Autodesk Fusion 360 part; units mm, degrees
sketch "Sketch2" plane through (0, 0, 0) normal (1, 0, 0) x (0, 1, 0)
  line L0 (-56.0607, 28.9615) -> (-14.2484, 28.9615)
  line L1 (-9.4019, 28.157) -> (-6.4108, 27.1358)
  arc A0 (-6.4108, 27.1358) -> (-8.6089, 30.3207) centre (-5.3607, 30.2115) ccw
  circle A1 centre (-5.3607, 30.2115) radius 2.75
  line L2 (-56.0607, 26.4615) -> (-14.2484, 26.4615)
  line L3 (-10.2097, 25.791) -> (-7.2185, 24.7698)
  arc A2 (-7.2185, 24.7698) -> (-11.1075, 30.4047) centre (-5.3607, 30.2115) ccw
  line L4 (-56.0607, 28.9615) -> (-56.0607, 26.4615)
  line L5 (-11.1075, 30.4047) -> (-11.1411, 29.4053)
  line L6 (-11.1411, 29.4053) -> (-8.6425, 29.3212)
  line L7 (-8.6425, 29.3212) -> (-8.6089, 30.3207)
  arc A3 (-9.4019, 28.157) -> (-14.2484, 28.9615) centre (-14.2484, 13.9615) ccw
  arc A4 (-10.2097, 25.791) -> (-14.2484, 26.4615) centre (-14.2484, 13.9615) ccw
  line L8 (14.6393, 52.3652) -> (14.6393, 9.6795) construction
  arc A5 (40.386, 30.4047) -> (36.497, 24.7698) centre (34.6393, 30.2115) ccw
  circle A6 centre (34.6393, 30.2115) radius 2.75
  line L9 (85.3393, 28.9615) -> (43.5269, 28.9615)
  line L10 (85.3393, 28.9615) -> (85.3393, 26.4615)
  arc A7 (43.5269, 28.9615) -> (38.6804, 28.157) centre (43.5269, 13.9615) ccw
  line L11 (40.386, 30.4047) -> (40.4196, 29.4053)
  arc A8 (37.8874, 30.3207) -> (35.6893, 27.1358) centre (34.6393, 30.2115) ccw
  line L12 (38.6804, 28.157) -> (35.6893, 27.1358)
  line L13 (40.4196, 29.4053) -> (37.921, 29.3212)
  line L14 (39.4882, 25.791) -> (36.497, 24.7698)
  line L15 (85.3393, 26.4615) -> (43.5269, 26.4615)
  arc A9 (43.5269, 26.4615) -> (39.4882, 25.791) centre (43.5269, 13.9615) ccw
  line L16 (37.921, 29.3212) -> (37.8874, 30.3207)
  dimension "d1" = 5.5
  dimension "d2" = 50.7
  dimension "d3" = 2.5
  dimension "d4" = 0
  dimension "d5" = 0.5
  dimension "d6" = 0
  dimension "d7" = 1
  dimension "d8" = 15
  dimension "d9" = 20
extrude "Extrude1" add sketch "Sketch2" along normal blind 101.4 contours L0 L1 A0 L2 L3 A2 L4 L5 L6 L7 A3 A4
sketch "Sketch1" plane through (0, 0, 28.9615) normal (0, 0, 1) x (-1, 0, 0)
  line L0 (0, 14.2484) -> (0, 56.0607)
  line L1 (0, 56.0607) -> (-101.4, 56.0607)
  line L2 (-101.4, 56.0607) -> (-101.4, 14.2484)
  line L3 (-101.4, 14.2484) -> (0, 14.2484)
  line L4 (0, 14.2484) -> (18.3824, 20.4527)
  line L5 (18.3824, 20.4527) -> (18.3824, -4.9808)
  line L6 (18.3824, -4.9808) -> (-17.5, -4.9808)
  line L7 (-17.5, -4.9808) -> (-17.5, 14.2484)
  line L8 (-40.8, 14.2484) -> (-40.8, 11.0057)
  line L9 (-40.8, 11.0057) -> (-40.8, -4.9808)
  line L10 (-40.8, -4.9808) -> (-60.6, -4.9808)
  line L11 (-60.6, -4.9808) -> (-60.6, 14.2484)
  line L12 (-83.9, 14.2484) -> (-83.9, -4.9808)
  line L13 (-83.9, -4.9808) -> (-134.9138, -4.9808)
  line L14 (-134.9138, -4.9808) -> (-127.3022, 20.8989)
  line L15 (-127.3022, 20.8989) -> (-101.4, 14.2484)
  circle A0 centre (-13.3, 46.0607) radius 3.6
  circle A1 centre (-63.3, 46.0607) radius 3.6
  circle A2 centre (-38.3, 37.0607) radius 3.6
  circle A3 centre (-88.3, 37.0607) radius 3.6
  arc A4 (0, 39.0607) -> (-17, 56.0607) centre (-17, 39.0607) ccw
  arc A5 (-84.4, 56.0607) -> (-101.4, 39.0607) centre (-84.4, 39.0607) ccw
  line L16 (0, 11.1411) -> (0, 8.6425)
  line L17 (-60.6, 11.6411) -> (-61.7689, 11.6411)
  line L18 (0, 11.6411) -> (-83.9, 11.6411)
  arc A6 (0, 11.6411) -> (0, 13.0607) centre (0, 12.3509) ccw
  line L19 (0, 13.0607) -> (0, 14.2484)
  line L20 (-83.9, 11.6411) -> (-104.4263, 11.6411)
  line L21 (-104.4263, 11.6411) -> (-104.4263, 15.0254)
  dimension "d25" = 17.5
  dimension "d26" = 17.5
  dimension "d27" = 23.3
  dimension "d28" = 23.3
  dimension "d37" = 7.2
  dimension "d40" = -25
  dimension "d41" = -9
  dimension "d42" = 13.3
  dimension "d43" = 10
  dimension "d44" = 17
  dimension "d45" = 17
  dimension "d78" = 0.5
extrude "Extrude2" cut sketch "Sketch1" along normal blind 10 and the other way blind 10 contours L4 L5 L6 L7 L18 A6 L19 | L0 L1 A4 | L1 L2 A5 | L8 L9 L10 L11 L18 | L12 L13 L14 L15 L20 L21 | A0 | A1 | A2 | A3
chamfer "Chamfer1" distance 2 angle 45 4 edges at (16.6564, -44.7589, 26.4615) (41.6564, -35.7589, 26.4615) (66.6564, -44.7589, 26.4615) (91.6564, -35.7589, 26.4615)
equation "d26 = d25"
equation "d27 = d28"
equation "d45 = d44"
equation "d2 = ( 101.4 / 2 ) * 1 mm"
equation "d4 = d4 / 2"
equation "d6 = d4"
Can you work these out from the model? Positions are in its coordinate system, mm. A direction names the side the tool comes from. Give positions to 0.01 mm unless a question says otherwise; leave off trailing zeros. Write each loop counter-clockwise with the first axis right and the second up, starting at its lowest first coordinate (ties: lowest second). Pieces come first, ordered by that corner, then holes. Notation, with made-up numbers: (45, -1) -> (60, -1) arc R17 cw to (60, 11) -> close; hole circle Ø6 at (66.25, -10.75). An arc over 180 degrees is marked (long way). Answer as a JSON object with one key per item and string values. Group by question number.
Item 1: We'd pull the mould along Z, two halves only. Please class faces 1 (the face through (72.087, -0.746, 33.641)), 2 (the face through (101.4, -26, 28)), 3 (the face through (72.09, -2.75, 32.15)): +Z half, -Z half, draft (parallel to the pull), parting line (faces both ways), or undercut.
Item 2: Suppose I cut it at A-A (x = 63.3). Please give me the cut outline in (y, z), plus the area to 3 significant figures.
Item 3: I'm going to push flat-ended pins straight in: P1, Ø3, axis at x = 77.5, y = -21.5, coming from the +Z side; P2, Ø1, axis at x = 50.5, y = -25.5, coming from the -Z side; P3, Ø2, axis at x = 91, z = 27.5, coming from the +Y side; P4, Ø1.5, axis at y = -7.5, z = 30.5, coming from the -X side. Where does each tip first touch, or does it pass through?
Item 4: Please list where these lines run through material, in increasing order: line 1 (X direction, y = -33, z = 27); line 2 (X direction, y = -46.5, z = 26.5); line 3 (X direction, y = -10, z = 30.5). Write a range as [from, to].
Item 5: Suppose I cut it at B-B (y = -23). Please give me the cut outline in (x, z), plus the area to 4 significant figures.
Item 6: Suppose I cut it at C-C (x = 88.3). Please give me the cut outline in (y, z), plus the area to 3 significant figures.
Item 7: For faces 4 (the face through (40.8, -3, 27.6)), 5 (the face through (9, -11.641, 27)), 6 (the face through (72.087, -7.927, 27.654)), which set-ups out of +Z, -Z, +X, -X, +Y, -Y let a thin tool reach every point of the face, with its end or its side?
Item 8: Suppose I cut it at D-D (x = 13.3). Please give me the cut outline in (y, z).
Findings:
{
 "1": {"face 1": "parting line", "face 2": "draft", "face 3": "undercut"},
 "2": {"outline": "(-56.06, 26.46) -> (-51.66, 26.46) -> (-49.66, 28.46) -> (-49.66, 28.96) -> (-56.06, 28.96) -> close; (-42.46, 28.46) -> (-40.46, 26.46) -> (-14.25, 26.46) arc R12.5 cw to (-10.21, 25.79) -> (-7.22, 24.77) arc R5.75 ccw (long way) to (-11.11, 30.4) -> (-11.14, 29.41) -> (-8.64, 29.32) -> (-8.61, 30.32) arc R3.25 cw (long way) to (-6.41, 27.14) -> (-9.4, 28.16) arc R15 ccw to (-14.25, 28.96) -> (-42.46, 28.96) -> close", "area": "161 mm²"},
 "3": {"P1": "stops at z = 28.96", "P2": "stops at z = 26.46", "P3": "stops at y = -11.64", "P4": "passes through"},
 "4": {"line 1": "x = [0, 35.28], [41.32, 85.28], [91.32, 101.4]", "line 2": "x = [1.71, 7.76], [18.84, 57.76], [68.84, 99.69]", "line 3": "x = [17.5, 40.8], [60.6, 83.9]"},
 "5": {"outline": "(0, 26.46) -> (101.4, 26.46) -> (101.4, 28.96) -> (0, 28.96) -> close", "area": "253.5 mm²"},
 "6": {"outline": "(-55.61, 26.46) -> (-42.66, 26.46) -> (-40.66, 28.46) -> (-40.66, 28.96) -> (-55.61, 28.96) -> close; (-33.46, 28.46) -> (-31.46, 26.46) -> (-14.25, 26.46) arc R12.5 cw to (-11.64, 26.19) -> (-11.64, 28.73) arc R15 ccw to (-14.25, 28.96) -> (-33.46, 28.96) -> close", "area": "88.0 mm²"},
 "7": {"face 4": "+Z, -Z, +Y", "face 5": "+Z, -Z, -X, +Y", "face 6": "+X, -X"},
 "8": {"outline": "(-55.65, 26.46) -> (-51.66, 26.46) -> (-49.66, 28.46) -> (-49.66, 28.96) -> (-55.65, 28.96) -> close; (-42.46, 28.46) -> (-40.46, 26.46) -> (-14.25, 26.46) arc R12.5 cw to (-11.64, 26.19) -> (-11.64, 28.73) arc R15 ccw to (-14.25, 28.96) -> (-42.46, 28.96) -> close"}
}
